Autodesk Inventor part; units mm, degrees
ref_plane "YZ Plane" through (0, 0, 0) normal (1, 0, 0) x (0, 1, 0)
ref_plane "XZ Plane" through (0, 0, 0) normal (0, 1, 0) x (-1, 0, 0)
ref_plane "XY Plane" through (0, 0, 0) normal (0, 0, 1) x (1, 0, 0)
sketch "Sketch1" plane through (0, 0, 0) normal (0, 1, 0) x (-1, 0, 0)
  line L0 (75, 8) -> (-75, 8)
  line L1 (-75, 8) -> (-75, -8)
  line L2 (-75, -8) -> (75, -8)
  line L3 (75, -8) -> (75, 8)
  line L4 (75, 8) -> (-75, -8) construction
  line L5 (-75, 8) -> (75, -8) construction
  line L6 (-75, 8) -> (-84, 8)
  line L7 (-84, 8) -> (-84, -8)
  line L8 (-84, -8) -> (-75, -8)
  line L9 (-75, -8) -> (-75, 8)
  line L10 (75, 8) -> (84, 8)
  line L11 (84, 8) -> (84, -8)
  line L12 (84, -8) -> (75, -8)
  line L13 (75, -8) -> (75, 8)
  point P0 (0, 0)
  dimension "d0" = 150
  dimension "d1" = 16
  dimension "d2" = 9
  dimension "d3" = 9
extrude "Extrusion1" add sketch "Sketch1" along normal blind 3
sketch "Sketch2" plane through (0, 3, 0) normal (0, 1, 0) x (1, 0, 0)
  line L0 (-70.5, 4.5) -> (70.5, 4.5)
  line L1 (70.5, 4.5) -> (70.5, -4.5)
  line L2 (70.5, -4.5) -> (-70.5, -4.5)
  line L3 (-70.5, -4.5) -> (-70.5, 4.5)
  line L4 (-70.5, 4.5) -> (70.5, -4.5) construction
  line L5 (70.5, 4.5) -> (-70.5, -4.5) construction
  circle A0 centre (-66.5, 0) radius 1.25
  circle A1 centre (-66.5, 0) radius 4
  circle A2 centre (66.5, 0) radius 1.25
  circle A3 centre (66.5, 0) radius 4
  point P0 (0, 0)
  dimension "d6" = 141
  dimension "d7" = 9
  dimension "d8" = 2.5
  dimension "d9" = 8
  dimension "d10" = 4
  dimension "d11" = 2.5
  dimension "d12" = 8
  dimension "d13" = 4
extrude "Extrusion2" add sketch "Sketch2" along normal blind 3 contours A1 | A3
sketch "Sketch3" plane through (0, 3, 0) normal (0, 1, 0) x (1, 0, 0)
  circle A0 centre (-66.5, 0) radius 1.25
  circle A1 centre (66.5, 0) radius 1.25
  point P0 (0, 0)
extrude "Extrusion3" cut sketch "Sketch3" against normal blind 3
sketch "Sketch4" plane through (0, 3, 0) normal (0, 1, 0) x (1, 0, 0)
  line L0 (-62.5, 4.7822) -> (62.5, 4.7822)
  line L1 (62.5, 4.7822) -> (62.5, 3.2178)
  line L2 (62.5, 3.2178) -> (-62.5, 3.2178)
  line L3 (-62.5, 3.2178) -> (-62.5, 4.7822)
  line L4 (-62.5, 4.7822) -> (62.5, 3.2178) construction
  line L5 (62.5, 4.7822) -> (-62.5, 3.2178) construction
  point P0 (0, 0)
  point P1 (0, 4)
extrude "Extrusion4" add sketch "Sketch4" along normal blind 3
sketch "Sketch5" plane through (0, 0, 0) normal (0, -1, 0) x (1, 0, 0)
  line L0 (84, -8) -> (-84, -8)
  line L1 (-84, 8) -> (-76, 8)
  line L2 (-76, 8) -> (-76, -8)
  line L3 (-76, -8) -> (-84, -8)
  line L4 (-84, -8) -> (-84, 8)
  line L5 (84, 8) -> (76, 8)
  line L6 (76, 8) -> (76, -8)
  line L7 (76, -8) -> (84, -8)
  line L8 (84, -8) -> (84, 8)
  point P0 (0, 0)
  dimension "d20" = 8
  dimension "d21" = 8
extrude "Extrusion5" add sketch "Sketch5" along normal blind 30
sketch "Sketch6" plane through (0, -30, 0) normal (0, -1, 0) x (1, 0, 0)
  line L0 (-84, 8) -> (-64, 8)
  line L1 (-64, 8) -> (-64, -8)
  line L2 (-64, -8) -> (-84, -8)
  line L3 (-84, -8) -> (-84, 8)
  point P0 (0, 0)
  dimension "d24" = 20
sketch "Sketch7" plane through (0, -30, 0) normal (0, -1, 0) x (1, 0, 0)
  line L0 (84, 8) -> (64, 8)
  line L1 (64, 8) -> (64, -8)
  line L2 (64, -8) -> (84, -8)
  line L3 (84, -8) -> (84, 8)
  point P0 (0, 0)
  dimension "d25" = 20
extrude "Extrusion6" add sketch "Sketch7" along normal blind 3
extrude "Extrusion7" add sketch "Sketch6" along normal blind 3
sketch "Sketch8" plane through (0, -33, 0) normal (0, -1, 0) x (1, 0, 0)
  line L0 (-84, -8) -> (-64, -8)
  line L1 (-76, -8) -> (-76, 8)
  line L2 (-64, 8) -> (-76, 8)
  line L3 (-64, -8) -> (-64, 8)
  line L4 (-76, -8) -> (-64, -8)
  circle A0 centre (-70, 0) radius 2.25
  point P0 (0, 0)
  dimension "d30" = 4.5
extrude "Extrusion8" cut sketch "Sketch8" against normal blind 3 contours A0
sketch "Sketch9" plane through (0, -33, 0) normal (0, -1, 0) x (1, 0, 0)
  line L0 (76, 8) -> (76, -8)
  line L1 (76, 8) -> (76, -8)
  line L2 (64, -8) -> (76, -8)
  line L3 (64, 8) -> (64, -8)
  line L4 (76, 8) -> (64, 8)
  circle A0 centre (70, 0) radius 2.25
  point P0 (0, 0)
  dimension "d33" = 4.5
extrude "Extrusion9" cut sketch "Sketch9" against normal blind 3 contours A0
sketch "Sketch11" plane through (0, 3, 0) normal (0, 1, 0) x (1, 0, 0)
  line L0 (-84, -8) -> (84, -8)
  line L1 (84, 8) -> (-84, 8)
  line L2 (-72.587, 8) -> (-74.587, 8)
  line L3 (-74.587, 8) -> (-74.587, -8)
  line L4 (-74.587, -8) -> (-72.587, -8)
  line L5 (-72.587, -8) -> (-72.587, 8)
  line L6 (-72.587, 8) -> (72.5136, 8)
  line L7 (72.5136, 8) -> (72.5136, 6.6306)
  line L8 (72.5136, 6.6306) -> (-72.587, 6.6306)
  line L9 (-72.587, 6.6306) -> (-72.587, 8)
  line L10 (72.5136, 8) -> (74.5136, 8)
  line L11 (74.5136, 8) -> (74.5136, -8)
  line L12 (74.5136, -8) -> (72.5136, -8)
  line L13 (72.5136, -8) -> (72.5136, 8)
  point P0 (0, 0)
  dimension "d38" = 2
  dimension "d39" = 2
extrude "Extrusion10" add sketch "Sketch11" along normal blind 13 contours L3 L1 L5 L0 | L13 L7 L1 L11 L0 | L5 L1 L7 L8
properties part number "montowanie kostek ark do rozdzielnicy"
Model file for the job. Use its own axes, mm. A direction names the side the tool comes from. Coordinates: 2 decimals unless noted, no trailing zeros. Write each loop counter-clockwise with the first axis right and the second up, starting at its lowest first coordinate (ties: lowest second). Pieces come first, ordered by that corner, then holes. Notation, with made-up numbers: (68.5, 67.5) - (76.5, 67.5) arc R19 ccw to (76.5, 103.5) - close; hole circle Ø5 at (14, -10). An arc over 180 degrees is marked (long way). Write each question's results on one line, items separated by ' | '. Start each with the question number.
1) Cut at A-A (y = -24.5). Write the cut outline in (x, z), then the cut area to 3 significant figures.
2) 3-axis set-ups, long thin cutter, end or side, ignore diameter. For faces 1 (the face through (76, -15, 0)), 2 (the face through (-74.587, 9, 0)), 3 (the face through (68, 6, 0)), 4 (the face through (-64, -31, 0)), 5 (the face through (-1, 4, -4.782)): which of +Z, -Z, +X, -X, +Y, -Y reach the whole face in a straight line?
3) Cut at C-C (y = 7.5). Write the cut outline in (x, z).
4) Cut at B-B (x = 48.5). Write the cut outline in (y, z).
5) Mould opens along Y. For faces 6 (the face through (73, -30, 0)), 7 (the face through (-0.4, 16, -7.7)), 8 (the face through (72.08, -31.52, -0.86)), 9 (the face through (-67, -30, 0)) say: pulls with the +Y half, pulls with the -Y half, needs draft (parallel to the pull), parting line crosses it, or undercut.
6) Flat gauge pins, fed straight in: P1, Ø1.5, axis at y = 7, z = 5.5, coming from the +X side; P2, Ø9, axis at x = -68.5, z = 0, coming from the +Y side; P3, Ø4.5, axis at x = 80, z = 2.5, coming from the +Y side; P4, Ø6.5, axis at y = 12, z = 3.5, coming from the -X side. Where does each tip first touch, or does it go through?
7) Probe line 1 along X through (y, z) = (2.05, 0); line 2 along X through (y, z) = (4.3, 0); line 3 along X through (y, z) = (-1, 1). List the from-to ranges inside material, lowest first. Write a range as from..to.
Returned:
1) outline: (-84, -8) - (-76, -8) - (-76, 8) - (-84, 8) - close; (76, -8) - (84, -8) - (84, 8) - (76, 8) - close | area: 256 mm^2
2) face 1: +Z, -Z | face 2: +Z, -Z, -X, +Y | face 3: +Z, +Y | face 4: +Z, -Z, -Y | face 5: +Y
3) outline: (-74.59, -8) - (74.51, -8) - (74.51, 8) - (72.51, 8) - (72.51, -6.63) - (-72.59, -6.63) - (-72.59, 8) - (-74.59, 8) - close
4) outline: (0, -8) - (16, -8) - (16, -6.63) - (3, -6.63) - (3, -4.78) - (6, -4.78) - (6, -3.22) - (3, -3.22) - (3, 8) - (0, 8) - close
5) face 6: undercut | face 7: pulls with the +Y half | face 8: needs draft | face 9: undercut
6) P1: x = 74.51 | P2: y = 16 | P3: y = 3 | P4: x = -74.59
7) line 1: -84..-67.75, -65.25..65.25, 67.75..84 | line 2: -74.59..-72.59, -70.5..-67.75, -65.25..-62.5, 62.5..65.25, 67.75..70.5, 72.51..74.51 | line 3: -84..-76, 76..84
